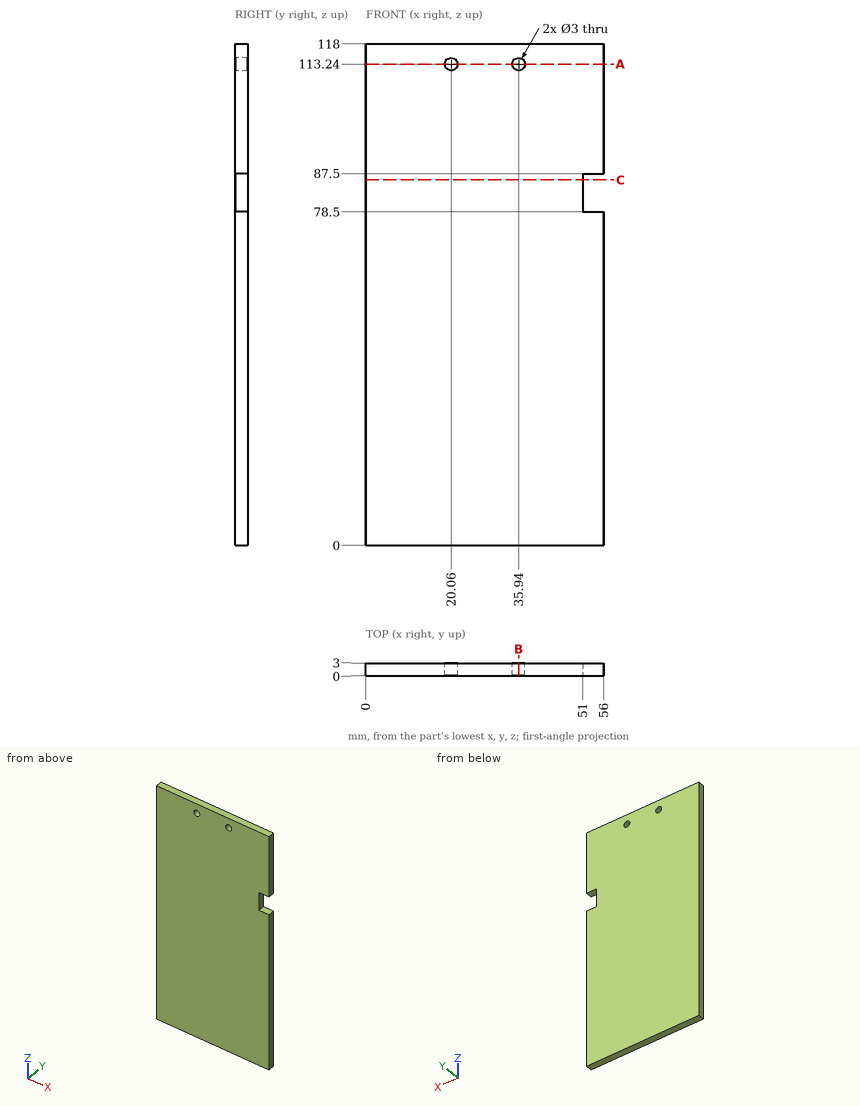
Check sheet for the drawn part. Datum: minimum x, y, z corner. Units: mm. Give positions to 0.01 mm unless a question says otherwise; leave off trailing zeros. Order: outer loops, then holes, each group sorted by start corner. A loop starts at its lowest first (then second) coordinate and runs counter-clockwise, first axis right, second up.
1. Sectioned sample at A-A (z = 113.24). Record the boundary of the cut face in (x, y).
Completed:
outline: (0, 0) - (18.56, 0) - (18.56, 3) - (0, 3) - close; (21.56, 0) - (34.44, 0) - (34.44, 3) - (21.56, 3) - close; (37.44, 0) - (56, 0) - (56, 3) - (37.44, 3) - close
2. Sectioned sample at B-B (x = 35.94). Record the boundary of the cut face in (y, z).
Completed:
outline: (0, 0) - (3, 0) - (3, 111.74) - (0, 111.74) - close; (0, 114.74) - (3, 114.74) - (3, 118) - (0, 118) - close
3. Sectioned sample at C-C (z = 86). Record the boundary of the cut face in (x, y), then the cut area to 3 significant figures.
Completed:
outline: (0, 0) - (51, 0) - (51, 3) - (0, 3) - close
area: 153 mm2
4. Scan lines: line 1 (X direction, y = 1.4, z = 113.24); line 2 (Z direction, x = 35.94, y = 1.65); line 3 (Z direction, x = 37, y = 2.8). Record each from-to range of solid material in increasing order.
Completed:
line 1: x = 0 to 18.56, 21.56 to 34.44, 37.44 to 56
line 2: z = 0 to 111.74, 114.74 to 118
line 3: z = 0 to 112.18, 114.3 to 118
